Build history of the part. All positions in model axes, mm. Face numbers are marked on the shaded views. A direction names the side the tool comes from. Round coordinates to 2 decimals unless told otherwise and drop trailing zeros. Order: outer loops, then holes, each group sorted by start corner. A loop starts at its lowest first (then second) coordinate and runs counter-clockwise, first axis right, second up. Notation, with made-up numbers: (4.25, 47) -> (14.25, 47) arc R29 cw to (14.25, 74) -> close; hole circle Ø11 at (-24, 53). An arc over 180 degrees is marked (long way). Answer as a JSON object with one key per item and string values.
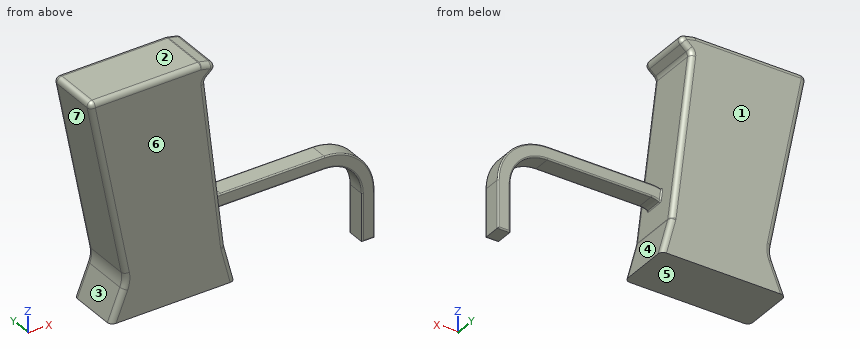
from build123d import *

# Parameters (mm, degrees)
BOSS_EXTRUDE1_DEPTH = 22
FILLET1_R           = 10
FILLET1_2_R         = 2
BOSS_EXTRUDE2_START = 6.25
BOSS_EXTRUDE2_DEPTH = 7.5
FILLET2_R           = 0.5


with BuildPart() as part:
    # Sketch1 → Boss-Extrude1 (new body)
    with BuildSketch(Plane(origin=(0, 0, 0), x_dir=(1, 0, 0), z_dir=(0, 1, 0))):
        Polygon((0, 0), (50, 0), (46.103209795, -15), (38.079497445, -82.972851485), (44.273841657, -88.266236279), (36.436917163, -90), (-8.563082837, -90), (6.103209795, -15), align=None)
    extrude(amount=BOSS_EXTRUDE1_DEPTH)

    # Fillet1
    fillet1_edges = [part.edges().sort_by_distance(p)[0] for p in [
        (6.103209795, 11, 15),
    ]]
    fillet(fillet1_edges, radius=FILLET1_R)

    # Fillet1 2
    fillet1_2_edges = [part.edges().sort_by_distance(p)[0] for p in [
        (40.35537941, 0, 89.133118139),
        (13.936917163, 0, 90),
        (-1.229936521, 0, 52.5),
        (3.051604897, 0, 7.5),
        (13.936917163, 22, 90),
        (46.103209795, 11, 15),
        (38.079497445, 11, 82.972851485),
        (44.273841657, 11, 88.266236279),
        (36.436917163, 11, 90),
        (-8.563082837, 11, 90),
        (40.35537941, 22, 89.133118139),
        (41.176669551, 22, 85.619543882),
        (42.09135362, 22, 48.986425743),
        (48.051604897, 22, 7.5),
        (3.051604897, 22, 7.5),
        (-1.229936521, 22, 52.5),
        (48.051604897, 0, 7.5),
        (42.09135362, 0, 48.986425743),
        (41.176669551, 0, 85.619543882),
    ]]
    fillet(fillet1_2_edges, radius=FILLET1_2_R)

    # Sketch2 → Boss-Extrude2 (add)
    with BuildSketch(Plane(origin=(0, 0, 0), x_dir=(1, 0, 0), z_dir=(0, 1, 0)).offset(BOSS_EXTRUDE2_START)):
        with BuildLine():
            Line((105, 7.5), (110, 7.5))
            Line((110, 7.5), (110, -11.5))
            ThreePointArc((110, -11.5), (104.142135624, -25.642135624), (90, -31.5))
            Line((90, -31.5), (48.388646792, -31.5))
            ThreePointArc((48.388646792, -31.5), (46.283857117, -31.321520216), (44.239173426, -30.791177667))
            Line((44.239173426, -30.791177667), (44.850427357, -25.612942101))
            ThreePointArc((44.850427357, -25.612942101), (46.564786293, -26.27485621), (48.388646792, -26.5))
            Line((48.388646792, -26.5), (90, -26.5))
            ThreePointArc((90, -26.5), (100.606601718, -22.106601718), (105, -11.5))
            Line((105, -11.5), (105, 7.5))
        make_face()
    extrude(amount=BOSS_EXTRUDE2_DEPTH)

    # Fillet2
    fillet2_edges = [part.edges().sort_by_distance(p)[0] for p in [
        (105, 6.25, 2),
        (100.606601718, 6.25, 22.106601718),
        (69.194323396, 6.25, 26.5),
        (46.564786293, 6.25, 26.27485621),
        (44.544800391, 6.25, 28.202059884),
        (44.850427357, 10, 25.612942101),
        (46.283857117, 6.25, 31.321520216),
        (44.239173426, 10, 30.791177667),
        (69.194323396, 6.25, 31.5),
        (104.142135624, 6.25, 25.642135624),
        (110, 6.25, 2),
        (107.5, 6.25, -7.5),
        (105, 13.75, 2),
        (100.606601718, 13.75, 22.106601718),
        (69.194323396, 13.75, 26.5),
        (46.564786293, 13.75, 26.27485621),
        (44.544800391, 13.75, 28.202059884),
        (46.283857117, 13.75, 31.321520216),
        (69.194323396, 13.75, 31.5),
        (104.142135624, 13.75, 25.642135624),
        (110, 13.75, 2),
        (107.5, 13.75, -7.5),
    ]]
    fillet(fillet2_edges, radius=FILLET2_R)


solid = part.part
1) Cut at C-C, the plane x = 74.5. Give the cut face in (y, z).
Checked values:
{"outline": "(6.25, 27) arc R0.5 ccw to (6.75, 26.5) -> (13.25, 26.5) arc R0.5 ccw to (13.75, 27) -> (13.75, 31) arc R0.5 ccw to (13.25, 31.5) -> (6.75, 31.5) arc R0.5 ccw to (6.25, 31) -> close"}
2) Which spindle directions (+Z, -Z, +X, -X, +Y, -Y) get a long thin tool onto all of the face, cutting with end or side? Do the marked faces 4, 5, 6 and 7. Say none if no direction does.
Checked values:
{"face 4": "+Y, -Y", "face 5": "-Z, -X, +Y, -Y", "face 6": "+Z, -Z, +X, -X, -Y", "face 7": "-X, +Y, -Y"}
3) Cut at A-A, the plane y = 4.25. Give the cut face in (x, z).
Checked values:
{"outline": "(-8.1, 87.62) -> (5.53, 17.93) arc R10 cw to (4.98, 12.24) -> (0, 0) -> (50, 0) -> (46.14, 14.87) arc R2 cw to (46.09, 15.14) -> (38.2, 81.91) arc R2 cw to (38.89, 83.67) -> (41.22, 85.66) arc R2 ccw to (40.36, 89.13) -> (36.65, 89.95) arc R2 ccw to (36.22, 90) -> (-6.13, 90) arc R2 ccw to start"}
4) Pull direction Z, two halves, no side cores. Call the marked faces 1, 2 and 3: pulls with the +Z half, pulls with the -Z half, needs draft (parallel to the pull), parting line crosses it, or undercut.
Checked values:
{"face 1": "needs draft", "face 2": "pulls with the +Z half", "face 3": "undercut"}
5) Cut at B-B, the plane x = 30.5. Give the cut face in (y, z).
Checked values:
{"outline": "(0, 0) -> (22, 0) -> (22, 88) arc R2 ccw to (20, 90) -> (2, 90) arc R2 ccw to (0, 88) -> close"}
6) Flat gauge pins, fed straight in: pin 1 Ø1.5 at (y, z) = (5, 22.5) entering from +X; pin 2 Ø10 at (x, y) = (56, 6.5) entering from +Z; pin 3 Ø2 at (x, y) = (64, 10) entering from -Z. Where does each tip first touch, or does it go through?
Checked values:
{"pin 1": "stops at x = 45.31", "pin 2": "stops at z = 31.5", "pin 3": "stops at z = 26.5"}
7) Probe L1, parallel to Z at x = 29, y = 7.5; L2, parallel to X at y = 10, z = 3.5; L3, parallel to X at y = 12, z = 10. List the from-to ranges inside material, lowest first. Write a range as from..to.
Checked values:
{"L1": "z = 0..90", "L2": "x = 1.42..49.09, 105..110", "L3": "x = 4.07..47.4, 105..110"}
